from build123d import *

# Parameters (mm, degrees)
SKETCH_W     = 130.707065
SKETCH_H     = 59.583364
SKETCH_W_2   = 30
SKETCH_H_2   = 39.583364
PAD_DEPTH    = 40
SKETCH001_R  = 9.347601
POCKET_DEPTH = 32


with BuildPart() as part:
    # Sketch → Pad (new body)
    with BuildSketch(Plane.XY):
        with Locations((-4.646459, 9.990193)):
            Rectangle(SKETCH_W, SKETCH_H)
        with Locations((-44.357391, 9.990193)):
            Rectangle(SKETCH_W_2, SKETCH_H_2, mode=Mode.SUBTRACT)
        with Locations((-5.023146, 10.351241)):
            Rectangle(SKETCH_W_2, SKETCH_H_2, mode=Mode.SUBTRACT)
        with Locations((35.101015, 9.990193)):
            Rectangle(SKETCH_W_2, SKETCH_H_2, mode=Mode.SUBTRACT)
    extrude(amount=PAD_DEPTH)

    # Sketch001 (on Face4 of Pad) → Pocket (cut)
    with BuildSketch(Plane(origin=(-69.999992, 0, 0), x_dir=(0, -1, 0), z_dir=(-1, 0, 0))):
        with Locations((-9.665334, 19.795595)):
            Circle(SKETCH001_R)
    extrude(amount=-POCKET_DEPTH, mode=Mode.SUBTRACT)


solid = part.part
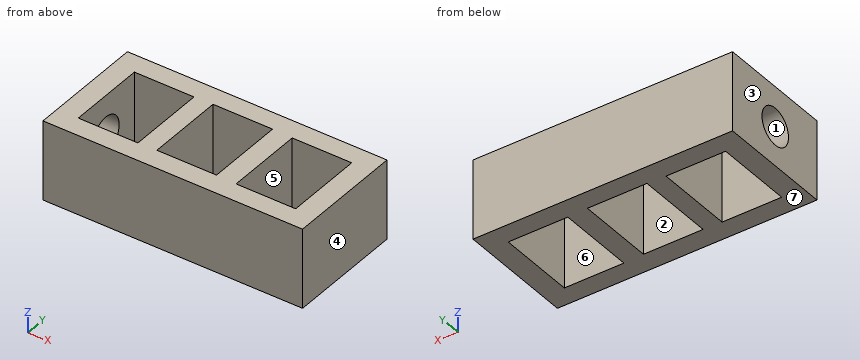
The listing builds one solid part. Answer for the finished solid, in the listing's coordinates (mm). Face numbers are marked on the shaded views. A direction names the side the tool comes from. Round coordinates to 2 decimals unless told otherwise and drop trailing zeros. Write each loop counter-clockwise with the first axis right and the second up, starting at its lowest first coordinate (ties: lowest second). Pieces come first, ordered by that corner, then holes. Notation, with made-up numbers: M 12.5,-31.75 L 36.5,-31.75 A13 ccw 36.5,-27.75 Z; hole C -14,34 d11. An arc over 180 degrees is marked long. Write each question's results on one line, items separated by ' | '. Start each with the question number.
Item 1: A flat-ended cylindrical pin translates along its axis: pin 1 Ø15 at (y, z) = (9.67, 19.8) entering from -X. Find the tip coordinate at first contact, or state that the pin passes through.
Item 2: Straight lines are drawn through the part: L1, parallel to X at y = -2, z = 33; L2, parallel to Y at x = -17, z = 36; L3, parallel to Y at x = 37.5, z = 16.5. For each, find the intervals that lie inside material, in ascending order. Write a range as [from, to].
Item 3: A cutting plane is placed at D-D on y = 10. Write down the section's boundary in (x, z), and give its area (3 significant figures).
Item 4: For the marked faces 1, 2 and 3, determine the directions among +Z, -Z, +X, -X, +Y, -Y from which every point of the face is accessible in a straight line to the end or side of a thin tool.
Item 5: A cutting plane is placed at C-C on y = -5. Write down the section's boundary in (x, z), and give its area (3 significant figures).
Item 6: For a pull along X with two mould halves and no side action, classify the marked faces 4, 5, 6 and 7 as pulls with the +X half, pulls with the -X half, needs draft (parallel to the pull), parting line crosses it, or undercut.
Item 7: A cutting plane is placed at A-A on z = 4. Write down the section's boundary in (x, y), and give its area (3 significant figures).
Item 8: A cutting plane is placed at B-B on x = -17.5. Write down the section's boundary in (y, z), and give its area (3 significant figures).
Check sheet entries:
1) pin 1: x = -29.36
2) L1: [-70, -59.36], [-29.36, -20.02], [9.98, 20.1], [50.1, 60.71] | L2: [-19.8, -9.44], [30.14, 39.78] | L3: [-19.8, -9.8], [29.78, 39.78]
3) outline: M -70,0 L -59.36,0 L -59.36,10.45 L -70,10.45 Z; M -70,29.14 L -59.36,29.14 L -59.36,40 L -70,40 Z; M -29.36,0 L -20.02,0 L -20.02,40 L -29.36,40 Z; M 9.98,0 L 20.1,0 L 20.1,40 L 9.98,40 Z; M 50.1,0 L 60.71,0 L 60.71,40 L 50.1,40 Z | area: 1,430 mm²
4) face 1: -X | face 2: +Z, -Z | face 3: +Z, -Z, -X, +Y, -Y
5) outline: M -70,0 L -59.36,0 L -59.36,40 L -70,40 Z; M -29.36,0 L -20.02,0 L -20.02,40 L -29.36,40 Z; M 9.98,0 L 20.1,0 L 20.1,40 L 9.98,40 Z; M 50.1,0 L 60.71,0 L 60.71,40 L 50.1,40 Z | area: 1,630 mm²
6) face 4: pulls with the +X half | face 5: undercut | face 6: undercut | face 7: needs draft
7) outline: M -70,-19.8 L 60.71,-19.8 L 60.71,39.78 L -70,39.78 Z; hole M -59.36,-9.8 L -29.36,-9.8 L -29.36,29.78 L -59.36,29.78 Z; hole M -20.02,-9.44 L 9.98,-9.44 L 9.98,30.14 L -20.02,30.14 Z; hole M 20.1,-9.8 L 50.1,-9.8 L 50.1,29.78 L 20.1,29.78 Z | area: 4,230 mm²
8) outline: M -19.8,0 L -9.44,0 L -9.44,40 L -19.8,40 Z; M 30.14,0 L 39.78,0 L 39.78,40 L 30.14,40 Z | area: 800 mm²
